Input: part model. Units: mm. Frame: model coordinates. A direction names the side the tool comes from. Coordinates: 2 decimals unless noted, no trailing zeros. Write each loop counter-clockwise with the first axis right and the second up, starting at its lowest first coordinate (ties: lowest second). Pieces come first, ordered by that corner, then holes. Notation, with made-up numbers: (-28.5, -13) - (27.5, -13) arc R24 cw to (27.5, 13) - close; hole circle Ø7 at (26, 38.5). An arc over 180 degrees is marked (long way). Put each result on its own line as item: value. Start each with the question number.
1. Pin query (flat end, axial travel): pin 1 (4 mm diameter, centred on x = -1, y = -160.5, fed in from -Z); pin 2 (1.2 mm diameter, centred on x = -1.625, y = -166, fed in from -Z); pin 3 (3 mm diameter, centred on y = -166, z = -3.9, fed in from +X). Return the tip coordinate at first contact, or that it passes through.
2. Pull-direction query (Y, two-part tool) for faces 3 (the cylindrical face through (-7.84, -170.4, -7.43)), 4 (the cylindrical face through (-2.419, -155.392, 1.479)), 5 (the cylindrical face through (1.805, -151.601, 1.521)), 6 (the flat face through (2.375, -161, 1)); classes: released by +Y, released by -Y, zero draft, split by the parting line, or undercut.
3. Cut plane B-B, the plane z = -4.5. Return loops of the section in (x, y) (3 decimals).
4. Cut plane A-A, the plane y = -166. Return loops of the section in (x, z) (3 decimals), and give its area (3 significant figures).
5. Cut plane C-C, the plane z = 0.25. Return loops of the section in (x, y) (3 decimals), and give its area (3 significant figures).
6. Cut plane D-D, the plane x = -6.5. Return loops of the section in (y, z), and give its area (3 significant figures).
7. Line query: line 1 (Y direction, x = -8.55, z = -3.9); line 2 (X direction, y = -156, z = 0.7) (3 decimals); line 3 (Y direction, x = -1.5, z = 2.75). Output: solid intervals per line, ascending.
8. Access query for faces 1 (the flat face through (-6, -151, 1)), 2 (the flat face through (-6.009, -164.8, -3.1)). Directions: +Z, -Z, +X, -X, +Y, -Y. A direction counts if a zero-diameter tool reaches every point of the face in a straight line with its end or side. Return the directions, or none.
Autodesk Inventor part; units mm, degrees
ref_plane "YZ Plane" through (0, 0, 0) normal (1, 0, 0) x (0, 1, 0)
ref_plane "XZ Plane" through (0, 0, 0) normal (0, 1, 0) x (-1, 0, 0)
ref_plane "XY Plane" through (0, 0, 0) normal (0, 0, 1) x (1, 0, 0)
ref_plane "Plano de trabajo1" through (0, 0, 0) normal (0, 0, 1) x (1, 0, 0)
sketch "Boceto1" plane through (0, 0, 0) normal (0, 0, 1) x (1, 0, 0)
  circle A0 centre (108.375, -226.9) radius 1.5
  circle A1 centre (108.375, -327.280446) radius 1.5
  line L0 (58.475, -218.4) -> (58.475, -213.4)
  line L1 (58.475, -213.4) -> (80.675, -213.4)
  line L2 (80.675, -213.4) -> (80.675, -218.4)
  line L3 (58.475, -218.4) -> (80.675, -218.4)
  line L4 (99.475, -248.4) -> (104.475, -248.4)
  line L5 (104.475, -248.4) -> (104.475, -268.4)
  line L6 (104.475, -268.4) -> (99.475, -268.4)
  line L7 (99.475, -330.5) -> (99.475, -268.4)
  line L8 (99.475, -330.5) -> (44.375, -330.5)
  line L9 (44.375, -330.5) -> (44.375, -223.4)
  line L10 (99.475, -223.4) -> (44.375, -223.4)
  line L11 (99.475, -248.4) -> (99.475, -223.4)
  line L12 (98.375, -209.4) -> (88.675, -209.4)
  line L13 (88.675, -209.4) -> (88.675, -176)
  line L14 (88.675, -176) -> (197.375, -176)
  line L15 (197.375, -176) -> (197.375, -326)
  line L16 (197.375, -326) -> (112.375, -326)
  line L17 (112.375, -326) -> (112.375, -223.4)
  arc A2 (112.375, -223.4) -> (98.375, -209.4) centre (98.375, -223.4) ccw
  line L18 (29.999359, -209.4) -> (29.999359, -326)
  line L19 (29.999359, -326) -> (20.625, -326)
  line L20 (20.625, -326) -> (20.625, -288)
  line L21 (20.625, -288) -> (9.375, -288)
  line L22 (9.375, -288) -> (9.375, -176)
  line L23 (9.375, -176) -> (20.625, -176)
  line L24 (20.625, -176) -> (20.625, -209.4)
  line L25 (20.625, -209.4) -> (29.999359, -209.4)
  circle A3 centre (69.375, -196) radius 1.6
  circle A4 centre (44.375, -196) radius 1.6
  circle A5 centre (215.275, -317.3) radius 1.5
  circle A6 centre (2.725, -309.3) radius 1.5
  circle A7 centre (2.725, -317.7) radius 1.5
  circle A8 centre (215.275, -311.6) radius 1.5
  line L26 (212.375, -161) -> (-5.625, -161)
  line L27 (-5.625, -161) -> (-5.625, -303)
  line L28 (-5.625, -303) -> (5.625, -303)
  line L29 (5.625, -303) -> (5.625, -306)
  line L30 (5.625, -306) -> (-1.875, -306)
  line L31 (-1.875, -306) -> (-1.875, -321)
  line L32 (-1.875, -321) -> (5.625, -321)
  line L33 (5.625, -321) -> (5.625, -341)
  line L34 (5.625, -341) -> (212.375, -341)
  line L35 (212.375, -341) -> (212.375, -321)
  line L36 (212.375, -321) -> (218.675, -321)
  line L37 (218.675, -321) -> (218.675, -307.9)
  line L38 (218.675, -307.9) -> (212.375, -307.9)
  line L39 (212.375, -307.9) -> (212.375, -161)
  circle A9 centre (143.025, -170) radius 1.5
  circle A10 centre (94.675, -170) radius 1.5
  circle A11 centre (191.375, -170) radius 1.5
  circle A12 centre (33.999359, -226.9) radius 1.5
  circle A13 centre (33.999359, -327.540446) radius 1.5
  circle A14 centre (143.025, -152) radius 1.5
  circle A15 centre (94.675, -152) radius 1.5
  circle A16 centre (191.375, -152) radius 1.5
  line L40 (-5.625, -161) -> (212.375, -161)
  line L41 (212.375, -161) -> (212.375, -14.1)
  line L42 (212.375, -14.1) -> (218.675, -14.1)
  line L43 (218.675, -14.1) -> (218.675, -1)
  line L44 (218.675, -1) -> (212.375, -1)
  line L45 (212.375, -1) -> (212.375, 19)
  line L46 (212.375, 19) -> (5.625, 19)
  line L47 (5.625, 19) -> (5.625, -1)
  line L48 (5.625, -1) -> (-1.875, -1)
  line L49 (-1.875, -1) -> (-1.875, -16)
  line L50 (-1.875, -16) -> (5.625, -16)
  line L51 (5.625, -16) -> (5.625, -19)
  line L52 (5.625, -19) -> (-5.625, -19)
  line L53 (-5.625, -19) -> (-5.625, -161)
  circle A17 centre (215.275, -4.7) radius 1.5
  circle A18 centre (2.725, -12.7) radius 1.5
  circle A19 centre (2.725, -4.3) radius 1.5
  circle A20 centre (215.275, -10.4) radius 1.5
  line L54 (91.875, 14.8) -> (91.875, -3.3)
  line L55 (91.875, -3.3) -> (83.875, -3.3)
  line L56 (83.875, -3.3) -> (83.875, 14.8)
  line L57 (83.875, 14.8) -> (91.875, 14.8)
  line L58 (163.175, 8.8) -> (163.175, 2.3)
  line L59 (163.175, 2.3) -> (156.675, 2.3)
  line L60 (156.675, 2.3) -> (156.675, 8.8)
  line L61 (156.675, 8.8) -> (163.175, 8.8)
  line L62 (145.075, 8.8) -> (145.075, 2.3)
  line L63 (145.075, 2.3) -> (138.575, 2.3)
  line L64 (138.575, 2.3) -> (138.575, 8.8)
  line L65 (138.575, 8.8) -> (145.075, 8.8)
  line L66 (102.375, 2.3) -> (102.375, 8.8)
  line L67 (102.375, 8.8) -> (108.875, 8.8)
  line L68 (108.875, 8.8) -> (108.875, 2.3)
  line L69 (108.875, 2.3) -> (102.375, 2.3)
  line L70 (184.675, 8.8) -> (184.675, 2.3)
  line L71 (184.675, 2.3) -> (178.175, 2.3)
  line L72 (178.175, 2.3) -> (178.175, 8.8)
  line L73 (178.175, 8.8) -> (184.675, 8.8)
  line L74 (126.975, 8.8) -> (126.975, 2.3)
  line L75 (126.975, 2.3) -> (120.475, 2.3)
  line L76 (120.475, 2.3) -> (120.475, 8.8)
  line L77 (120.475, 8.8) -> (126.975, 8.8)
  circle A21 centre (44.375, -126) radius 1.6
  circle A22 centre (69.375, -126) radius 1.6
  line L78 (20.625, -146) -> (9.375, -146)
  line L79 (9.375, -146) -> (9.375, -34)
  line L80 (9.375, -34) -> (20.625, -34)
  line L81 (20.625, -34) -> (20.625, 4)
  line L82 (20.625, 4) -> (49.475, 4)
  line L83 (49.475, 4) -> (49.475, -112.6)
  line L84 (49.475, -112.6) -> (20.625, -112.6)
  line L85 (20.625, -112.6) -> (20.625, -146)
  line L86 (88.675, -146) -> (88.675, -10.3)
  line L87 (88.675, -10.3) -> (197.375, -10.3)
  line L88 (197.375, -10.3) -> (197.375, -146)
  line L89 (197.375, -146) -> (88.675, -146)
  line L90 (220.675, 19) -> (220.675, -161)
  line L91 (-7.625, 19) -> (-7.625, -161)
  line L92 (212.875, -14.6) -> (212.875, -161)
  line L93 (-6.125, -161) -> (-6.125, -18.5)
  line L94 (-7.625, -161) -> (2.375, -161)
  line L95 (2.375, -161) -> (2.375, -171)
  line L96 (2.375, -171) -> (-9.625, -171)
  line L97 (-9.625, -171) -> (-9.625, -151)
  line L98 (-9.625, -151) -> (2.375, -151)
  line L99 (2.375, -151) -> (2.375, -171)
  line L100 (2.375, -151) -> (-1.625, -151)
  line L101 (-1.625, -151) -> (-1.625, -171)
  line L102 (2.375, -151) -> (2.375, -156)
  line L103 (2.375, -156) -> (-1.625, -156)
  line L104 (2.375, -171) -> (2.375, -166)
  line L105 (2.375, -166) -> (-1.625, -166)
  circle A23 centre (-1.625, -156) radius 1
  circle A24 centre (-1.625, -166) radius 1
  line L106 (-7.625, -161) -> (-6.125, -161)
  line L107 (-6.125, -18.5) -> (5.125, -18.5)
  line L108 (5.125, -18.5) -> (5.125, -16.5)
  line L109 (5.125, -16.5) -> (-2.375, -16.5)
  line L110 (-2.375, -16.5) -> (-2.375, -0.5)
  line L111 (-2.375, -0.5) -> (5.125, -0.5)
  line L112 (5.125, -0.5) -> (5.125, 19.5)
  line L113 (5.125, 19.5) -> (212.875, 19.5)
  line L114 (212.875, 19.5) -> (212.875, -0.5)
  line L115 (212.875, -0.5) -> (219.175, -0.5)
  line L116 (219.175, -0.5) -> (219.175, -14.6)
  line L117 (219.175, -14.6) -> (212.875, -14.6)
  line L118 (212.875, -161) -> (220.675, -161)
  arc A25 (220.675, 19) -> (218.675, 21) centre (218.675, 19) ccw
  line L119 (218.675, 21) -> (-5.625, 21)
  arc A26 (-5.625, 21) -> (-7.625, 19) centre (-5.625, 19) ccw
  circle A27 centre (216.675, -156) radius 1.5
  point P0 (0, 0)
  dimension "d0" = 10
  dimension "d1" = 10
  dimension "d2" = 12
  dimension "d3" = 20
  dimension "d4" = 4
  dimension "d5" = 5
  dimension "d6" = 5
  dimension "d7" = 2
  dimension "d8" = 2
extrude "Extrusión1" add sketch "Boceto1" along normal blind 3 contours L95 L105 A24 L101 L26 | L26 L101 A23 L103 L99 | L101 A24 L96 L27 L26 | L26 L53 L98 L101 A23 | L95 L96 L101 A24 L105 | L103 A23 L101 L98 L99 | L94 L93 L98 L53 | L27 L96 L97 L98 L91 L94 | L94 L91 L98 L93
sketch "Boceto2" plane through (0, 0, 0) normal (0, 0, -1) x (-1, 0, 0)
  line L0 (7.625, 19) -> (7.625, -161)
  line L1 (-2.375, -151) -> (9.625, -151)
  line L2 (-2.375, -171) -> (-2.375, -151)
  line L3 (9.625, -171) -> (-2.375, -171)
  line L4 (9.625, -151) -> (9.625, -171)
  circle A0 centre (1.625, -166) radius 1
  circle A1 centre (1.625, -156) radius 1
  line L5 (-14.191374, -161) -> (6.008626, -161)
  line L6 (7.625, 19) -> (7.625, -161)
  arc A2 (7.625, 19) -> (5.625, 21) centre (5.625, 19) ccw
  line L7 (5.625, 21) -> (-218.675, 21)
  arc A3 (-218.675, 21) -> (-220.675, 19) centre (-218.675, 19) ccw
  line L8 (-220.675, 19) -> (-220.675, -161)
  line L9 (-222.291374, -161) -> (-209.991374, -161)
  line L10 (-208.375, -161) -> (-208.375, 9.8)
  line L11 (-208.375, 9.8) -> (-12.575, 9.8)
  line L12 (-12.575, 9.8) -> (-12.575, -161)
  circle A4 centre (-215.275, -4.7) radius 1.2
  circle A5 centre (-2.725, -4.3) radius 1.2
  circle A6 centre (-2.725, -12.7) radius 1.2
  circle A7 centre (-215.275, -10.4) radius 1.2
  line L13 (6.008626, -161) -> (-14.191374, -161)
  line L14 (-14.191374, -161) -> (-14.191374, -337)
  line L15 (-14.191374, -337) -> (-209.991374, -337)
  line L16 (-209.991374, -337) -> (-209.991374, -161)
  line L17 (-209.991374, -161) -> (-222.291374, -161)
  line L18 (-222.291374, -161) -> (-222.291374, -346.2)
  arc A8 (-222.291374, -346.2) -> (-220.291374, -348.2) centre (-220.291374, -346.2) ccw
  line L19 (4.008626, -348.2) -> (-220.291374, -348.2)
  arc A9 (4.008626, -348.2) -> (6.008626, -346.2) centre (4.008626, -346.2) ccw
  line L20 (6.008626, -161) -> (6.008626, -346.2)
  circle A10 centre (-216.891374, -311.6) radius 1.2
  circle A11 centre (-4.341374, -309.3) radius 1.2
  circle A12 centre (-4.341374, -317.7) radius 1.2
  circle A13 centre (-216.891374, -317.3) radius 1.2
  line L21 (-2.375, -151) -> (9.625, -151)
  line L22 (9.625, -151) -> (9.625, -171)
  line L23 (9.625, -171) -> (-2.375, -171)
  line L24 (-2.375, -171) -> (-2.375, -151)
  circle A14 centre (1.625, -166) radius 1
  circle A15 centre (1.625, -156) radius 1
  point P0 (0, 0)
  point P1 (6.098425, -151)
  point P2 (7.625, -171)
  point P3 (6.008626, -171)
sketch "Boceto2 outline for Extrusión2" plane through (0, 0, 0) normal (0, 0, -1) x (-1, 0, 0)
  line L0 (6.008626, -161) -> (6.008626, -171)
  line L1 (6.098425, -151) -> (6.008626, -161)
  line L2 (9.625, -151) -> (6.098425, -151)
  line L3 (9.625, -171) -> (9.625, -151)
  line L4 (6.008626, -171) -> (9.625, -171)
extrude "Extrusión2" add sketch "Boceto2 outline for Extrusión2" along normal blind 8
fillet "Empalme1" radius 2 1 edges at (-9.625, -161, 3)
sketch "Boceto4" plane through (-9.625, -171, -8) normal (-1, 0, 0) x (0, 0, 1)
  line L0 (9, 20) -> (9, 0)
  line L1 (0, 20) -> (9, 20)
  line L2 (0, 0) -> (0, 20)
  line L3 (0, 0) -> (9, 0)
  line L4 (4.1, 262) -> (4.1, -242)
  line L5 (4.1, 20) -> (4.1, 15)
  circle A0 centre (4.1, 15) radius 1
  line L6 (8, 0) -> (0, 0)
  line L7 (4.1, 0) -> (4.1, 5)
  circle A1 centre (4.1, 5) radius 1
  point P0 (8, 171)
  dimension "d14" = 5
  dimension "d15" = 2
  dimension "d16" = 5
  dimension "d17" = 2
hole "Agujero1" at (-9.625, -166, -3.9) at (-9.625, -156, -3.9) direction (1, 0, 0) diameter 2.4 end through all
fillet "Empalme2" radius 2 4 edges at (-7.8617, -151, -8) (-7.8168, -171, -8) (2.375, -151, 1.5) (2.375, -171, 1.5)
properties part number "Union abajo"
Report:
1. pin 1: stops at z = 0
1. pin 2: passes through
1. pin 3: stops at x = -6.01
2. face 3: released by -Y
2. face 4: undercut
2. face 5: released by +Y
2. face 6: zero draft
3. outline: (-9.625, -171) - (-6.009, -171) - (-6.009, -167.039) - (-9.625, -167.039) - close; (-9.625, -164.961) - (-6.009, -164.961) - (-6.009, -161) - (-6.044, -157.039) - (-9.625, -157.039) - close; (-9.625, -154.961) - (-6.063, -154.961) - (-6.098, -151) - (-9.625, -151) - close
4. outline: (-9.625, -8) - (-6.009, -8) - (-6.009, -5.1) - (-9.625, -5.1) - close; (-9.625, -2.7) - (-6.009, -2.7) - (-6.009, 0) - (-2.625, 0) - (-2.625, 3) - (-7.625, 3) arc R2 ccw to (-9.625, 1) - close; (-0.625, 0) - (2.375, 0) - (2.375, 3) - (-0.625, 3) - close
4. area: 49.4 mm^2
5. outline: (-9.625, -171) - (0.375, -171) arc R2 ccw to (2.375, -169) - (2.375, -153) arc R2 ccw to (0.375, -151) - (-9.625, -151) - close; hole circle Ø2 at (-1.625, -166); hole circle Ø2 at (-1.625, -156)
5. area: 232 mm^2
6. outline: (-171, -6) arc R2 ccw to (-169, -8) - (-153, -8) arc R2 ccw to (-151, -6) - (-151, 3) - (-171, 3) - close; hole circle Ø2.4 at (-166, -3.9); hole circle Ø2.4 at (-156, -3.9)
6. area: 209 mm^2
7. line 1: y = -171 to -167.2, -164.8 to -157.2, -154.8 to -151
7. line 2: x = -9.625 to -2.625, -0.625 to 2.375
7. line 3: y = -171 to -166.99, -165.01 to -156.99, -155.01 to -151
8. face 1: +Z, -Z, +X, -X, +Y
8. face 2: -Z, +X, +Y, -Y
